Source: CAD feature listing. Evaluate the final solid. Frame: model axes, mm. Coordinates: 2 decimals unless noted, no trailing zeros. Write each loop counter-clockwise with the first axis right and the second up, starting at its lowest first coordinate (ties: lowest second). Pieces come first, ordered by that corner, then holes. Notation, with made-up numbers: M 20,20.5 L 78,20.5 A30 cw 78,59.5 Z; hole C 28.25,-36.75 d9. An arc over 180 degrees is marked long. One line per item, written item: value. Start each with the question number.
Item 1: Cut plane C-C, the plane x = 31. Output: boundary loops of the cut face in (y, z) (3 decimals), then the cut area to 3 significant figures.
Item 2: Ray query, L1, parallel to Z at x = 75.55, y = 2.45; L2, parallel to X at y = 2, z = -11.3; L3, parallel to X at y = 2.3, z = -19.05. Return the intervals inside material, ascending. Write a range as from..to.
Item 3: Cut plane B-B, the plane z = -26.8. Output: boundary loops of the cut face in (x, y) (3 decimals).
Item 4: Cut plane A-A, the plane z = -6.35. Output: boundary loops of the cut face in (x, y) (3 decimals).
Item 5: Cut plane D-D, the plane x = 79. Output: boundary loops of the cut face in (y, z) (3 decimals), then the cut area to 3 significant figures.
```python
from build123d import *

# Parameters (mm, degrees)
SKETCH1_W           = 80
SKETCH1_H           = 38.1
SKETCH1_R           = 6.5
SKETCH1_R_2         = 1.75
BOSS_EXTRUDE1_DEPTH = 3.175
SKETCH2_W           = 80
SKETCH2_H           = 6.35
BOSS_EXTRUDE2_DEPTH = 3.175


with BuildPart() as part:
    # Sketch1 → Boss-Extrude1 (new body)
    with BuildSketch(Plane(origin=(0, 0, 0), x_dir=(1, 0, 0), z_dir=(0, 1, 0))):
        with Locations((62.55, 19.05)):
            Rectangle(SKETCH1_W, SKETCH1_H)
        with Locations(Location((82.55, 19.05, 0), (0, 0, 270))):
            Circle(SKETCH1_R, mode=Mode.SUBTRACT)
        with Locations(Location((75.55, 34.55, 0), (0, 0, 270))):
            Circle(SKETCH1_R_2, mode=Mode.SUBTRACT)
        with Locations(Location((88.973393759, 26.8, 0), (0, 0, 270))):
            Circle(SKETCH1_R_2, mode=Mode.SUBTRACT)
        with Locations(Location((88.973393759, 11.3, 0), (0, 0, 270))):
            Circle(SKETCH1_R_2, mode=Mode.SUBTRACT)
        with Locations(Location((75.55, 3.55, 0), (0, 0, 270))):
            Circle(SKETCH1_R_2, mode=Mode.SUBTRACT)
        with Locations(Location((62.126606241, 11.3, 0), (0, 0, 270))):
            Circle(SKETCH1_R_2, mode=Mode.SUBTRACT)
        with Locations(Location((62.126606241, 26.8, 0), (0, 0, 270))):
            Circle(SKETCH1_R_2, mode=Mode.SUBTRACT)
        with BuildLine():
            Line((29.55, 29.5), (34.55, 29.5))
            ThreePointArc((34.55, 29.5), (36.8, 31.75), (34.55, 34))
            Line((34.55, 34), (29.55, 34))
            ThreePointArc((29.55, 34), (27.3, 31.75), (29.55, 29.5))
        make_face(mode=Mode.SUBTRACT)
        with BuildLine():
            Line((29.55, 4.1), (34.55, 4.1))
            ThreePointArc((34.55, 4.1), (36.8, 6.35), (34.55, 8.6))
            Line((34.55, 8.6), (29.55, 8.6))
            ThreePointArc((29.55, 8.6), (27.3, 6.35), (29.55, 4.1))
        make_face(mode=Mode.SUBTRACT)
    extrude(amount=BOSS_EXTRUDE1_DEPTH)

    # Sketch2 → Boss-Extrude2 (add)
    with BuildSketch(Plane(origin=(0, 3.175, 0), x_dir=(1, 0, 0), z_dir=(0, 1, 0))):
        with Locations((62.55, 41.275)):
            Rectangle(SKETCH2_W, SKETCH2_H)
        with Locations((62.55, -3.175)):
            Rectangle(SKETCH2_W, SKETCH2_H)
    extrude(amount=-BOSS_EXTRUDE2_DEPTH)


solid = part.part
```
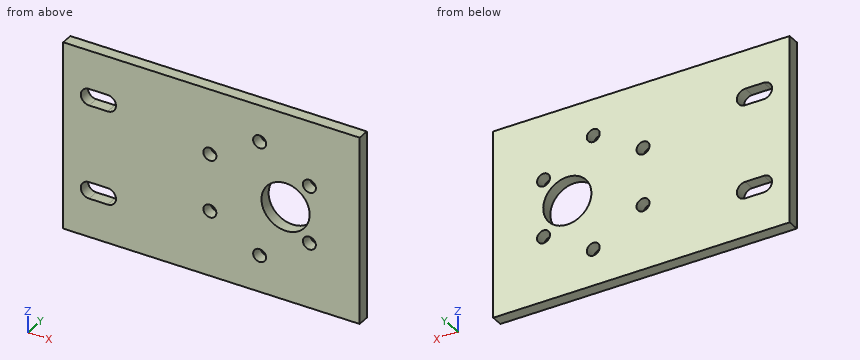
From the geometry:
1. outline: M 0,-44.45 L 3.175,-44.45 L 3.175,-34 L 0,-34 Z; M 0,-29.5 L 3.175,-29.5 L 3.175,-8.6 L 0,-8.6 Z; M 0,-4.1 L 3.175,-4.1 L 3.175,6.35 L 0,6.35 Z
1. area: 133 mm²
2. L1: z = -44.45..-36.3, -32.8..-5.3, -1.8..6.35
2. L2: x = 22.55..60.38, 63.88..87.22, 90.72..102.55
2. L3: x = 22.55..76.05, 89.05..102.55
3. outline: M 22.55,0 L 60.377,0 L 60.377,3.175 L 22.55,3.175 Z; M 63.877,0 L 87.223,0 L 87.223,3.175 L 63.877,3.175 Z; M 90.723,0 L 102.55,0 L 102.55,3.175 L 90.723,3.175 Z
4. outline: M 22.55,0 L 27.3,0 L 27.3,3.175 L 22.55,3.175 Z; M 36.8,0 L 102.55,0 L 102.55,3.175 L 36.8,3.175 Z
5. outline: M 0,-44.45 L 3.175,-44.45 L 3.175,-24.495 L 0,-24.495 Z; M 0,-13.605 L 3.175,-13.605 L 3.175,6.35 L 0,6.35 Z
5. area: 127 mm²
